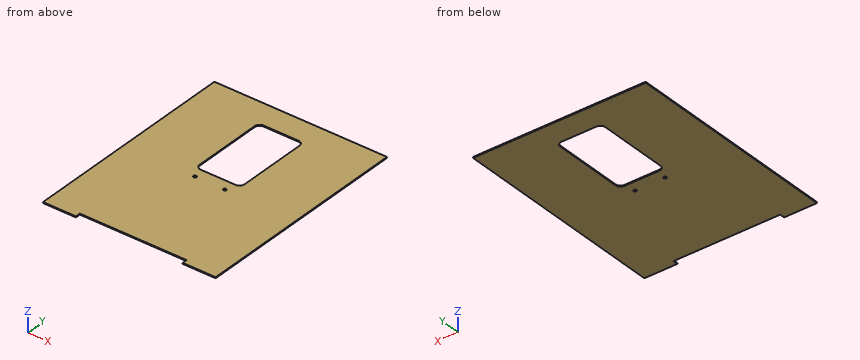
from build123d import *

# Parameters (mm, degrees)
T_LE_DE_BASE_PLI_E1_DEPTH = 1
ESQUISSE2_R               = 1.5
ESQUISSE2_W               = 45
ESQUISSE2_H               = 80
ENL_V_MAT_EXTRU_1_DEPTH   = 1
CONG_1_R                  = 5


# Sheet-metal steps are written as plain solids
with BuildPart() as part:
    # Esquisse1 → Tôle de base pliée1 (new body)
    with BuildSketch(Plane.XY):
        Polygon((53.5, 0), (86.5, 0), (86.5, 218), (-86.5, 218), (-86.5, 0), (-53.5, 0), (-53.5, 5), (53.5, 5), align=None)
    extrude(amount=-T_LE_DE_BASE_PLI_E1_DEPTH)

    # Esquisse2 → Enlèv. mat.-Extru.1 (cut)
    with BuildSketch(Plane.XY):
        with Locations((-15, 102.5)):
            Circle(ESQUISSE2_R)
        with Locations(Location((15, 102.5, 0), (0, 0, 180))):
            Circle(ESQUISSE2_R)
        with Locations((0, 153)):
            Rectangle(ESQUISSE2_W, ESQUISSE2_H)
    extrude(amount=-ENL_V_MAT_EXTRU_1_DEPTH, mode=Mode.SUBTRACT)

    # Congé1
    cong_1_edges = [part.edges().sort_by_distance(p)[0] for p in [
        (-22.5, 113, -0.5),
        (-22.5, 193, -0.5),
        (22.5, 193, -0.5),
        (22.5, 113, -0.5),
    ]]
    fillet(cong_1_edges, radius=CONG_1_R)


solid = part.part
The model under review builds one solid part; all positions refer to its coordinate system, in mm. Round coordinates to 2 decimals unless told otherwise and drop trailing zeros. Loops run counter-clockwise (first coordinate to the right, second up) from the corner with the lowest first, then second, coordinate; pieces in that order, holes last. Notation, with made-up numbers: (-32, 60.25) -> (19, 60.25) arc R34 cw to (19, 97.25) -> close; hole circle Ø4 at (87.25, 83.5). An arc over 180 degrees is marked (long way). Answer as CSV lines item,"result".
1) For P1, Ø0.5, axis at x = -4, z = -0.5, coming from the -Y side; P2, Ø6, axis at x = 2, y = 81, coming from the +Z side; P3, Ø2.5, axis at x = 15, y = 102.5, coming from the -Z side, all flat-tipped, find the tip position at first contact; note any pin that passes through.
Geometry results:
P1,"stops at y = 5"
P2,"stops at z = 0"
P3,"passes through"
2) Add section B-B on x = -8. Write out the cut boundary in (y, z).
Geometry results:
outline,"(5, -1) -> (113, -1) -> (113, 0) -> (5, 0) -> close; (193, -1) -> (218, -1) -> (218, 0) -> (193, 0) -> close"
3) To check wall thickness, follow line 1 along X through (y, z) = (102.5, -0.25); line 2 along Y through (x, z) = (15, -0.2); line 3 along Y through (x, z) = (-14.5, -0.5). State the ranges of each line that lie inside material, in increasing order. Write a range as from..to.
Geometry results:
line 1,"x = -86.5..-16.5, -13.5..13.5, 16.5..86.5"
line 2,"y = 5..101, 104..113, 193..218"
line 3,"y = 5..101.09, 103.91..113, 193..218"
4) Add section A-A on y = 137. Write out the cut boundary in (x, z), plus the area to 3 significant figures.
Geometry results:
outline,"(-86.5, -1) -> (-22.5, -1) -> (-22.5, 0) -> (-86.5, 0) -> close; (22.5, -1) -> (86.5, -1) -> (86.5, 0) -> (22.5, 0) -> close"
area,"128 mm²"
5) Add section C-C on z = -0.35. Write out the cut boundary in (x, y).
Geometry results:
outline,"(-86.5, 0) -> (-53.5, 0) -> (-53.5, 5) -> (53.5, 5) -> (53.5, 0) -> (86.5, 0) -> (86.5, 218) -> (-86.5, 218) -> close; hole (-22.5, 118) arc R5 ccw to (-17.5, 113) -> (17.5, 113) arc R5 ccw to (22.5, 118) -> (22.5, 188) arc R5 ccw to (17.5, 193) -> (-17.5, 193) arc R5 ccw to (-22.5, 188) -> close; hole circle Ø3 at (-15, 102.5); hole circle Ø3 at (15, 102.5)"
6) Add section D-D on x = -35. Write out the cut boundary in (y, z).
Geometry results:
outline,"(5, -1) -> (218, -1) -> (218, 0) -> (5, 0) -> close"
